from build123d import *

# Parameters (mm, degrees)
F0_W      = 160.02
F0_H      = 160.02
F1_DEPTH  = 61.214
F3_DEPTH  = 58.42
F4_R      = 3.937
F5_DEPTH  = 6.35
F7_DEPTH  = 6.35
F8_R      = 1.7018
F9_DEPTH  = 6.35
F11_R     = 6.35
F12_DEPTH = 6.35
F13_R     = 3.175
F14_DEPTH = 6.35
F15_R     = 6.35
F16_DEPTH = 6.35
F17_R     = 6.35
F18_DEPTH = 6.35
F19_R     = 3.81
F20_DEPTH = 6.35
F23_DEPTH = 6.35
F24_W     = 12.7
F24_H     = 12.7
F24_R     = 1.8288
F25_DEPTH = 6.35


with BuildPart() as f1:
    # F0 (on Top) → F1 (new body)
    with BuildSketch(Plane.XY):
        with Locations((80.01, 80.01)):
            Rectangle(F0_W, F0_H)
    extrude(amount=-F1_DEPTH)

    # F2 (on face) → F3 (cut)
    with BuildSketch(Plane.XY):
        Polygon((142.24, 154.305), (17.78, 154.305), (17.78, 135.89), (5.08, 135.89), (5.08, 24.13), (17.78, 24.13), (17.78, 5.715), (142.24, 5.715), (142.24, 24.13), (154.94, 24.13), (154.94, 135.89), (142.24, 135.89), align=None)
    extrude(amount=-F3_DEPTH, mode=Mode.SUBTRACT)

    # F4 (on face) → F5 (cut)
    with BuildSketch(Plane.XZ):
        with Locations((32.7025, -45.974)):
            Circle(F4_R)
        with Locations((127.3429, -45.974)):
            Circle(F4_R)
    extrude(amount=-F5_DEPTH, mode=Mode.SUBTRACT)

    # F6 (on face) → F7 (cut)
    with BuildSketch(Plane.XZ):
        with BuildLine():
            Line((81.1022, -35.9791), (61.1378, -35.9791))
            ThreePointArc((61.1378, -35.9791), (58.318, -37.1471), (57.15, -39.9669))
            Line((57.15, -39.9669), (57.15, -51.9811))
            ThreePointArc((57.15, -51.9811), (58.318, -54.8009), (61.1378, -55.9689))
            Line((61.1378, -55.9689), (81.1022, -55.9689))
            ThreePointArc((81.1022, -55.9689), (83.922, -54.8009), (85.09, -51.9811))
            Line((85.09, -51.9811), (85.09, -39.9669))
            ThreePointArc((85.09, -39.9669), (83.922, -37.1471), (81.1022, -35.9791))
        make_face()
    extrude(amount=-F7_DEPTH, mode=Mode.SUBTRACT)

    # F8 (on face) → F9 (cut)
    with BuildSketch(Plane.XZ):
        with Locations((51.1302, -45.974)):
            Circle(F8_R)
        with Locations((91.0082, -45.974)):
            Circle(F8_R)
    extrude(amount=-F9_DEPTH, mode=Mode.SUBTRACT)

    # F11 (on face) → F12 (cut)
    with BuildSketch(Plane.XZ):
        with Locations((32.6898, -26.924)):
            Circle(F11_R)
        with Locations((127.3302, -26.924)):
            Circle(F11_R)
    extrude(amount=-F12_DEPTH, mode=Mode.SUBTRACT)

    # F13 (on face) → F14 (cut)
    with BuildSketch(Plane.XZ):
        with Locations((32.6898, -10.414)):
            Circle(F13_R)
        with Locations((127.3302, -10.414)):
            Circle(F13_R)
    extrude(amount=-F14_DEPTH, mode=Mode.SUBTRACT)

    # F15 (on face) → F16 (cut)
    with BuildSketch(Plane.XZ):
        with Locations((71.12, -16.764)):
            Circle(F15_R)
    extrude(amount=-F16_DEPTH, mode=Mode.SUBTRACT)

    # F17 (on face) → F18 (cut)
    with BuildSketch(Plane.XZ):
        with Locations((106.68, -26.924)):
            Circle(F17_R)
    extrude(amount=-F18_DEPTH, mode=Mode.SUBTRACT)

    # F19 (on face) → F20 (cut)
    with BuildSketch(Plane.XZ):
        with Locations((106.68, -10.414)):
            Circle(F19_R)
    extrude(amount=-F20_DEPTH, mode=Mode.SUBTRACT)

    # F22 (on face) → F23 (cut)
    with BuildSketch(Plane(origin=(0, 160.02, 0), x_dir=(-1, 0, 0), z_dir=(0, 1, 0))):
        with BuildLine():
            ThreePointArc((-139.419261, -17.800688), (-140.943261, -19.324688), (-139.419261, -20.848688))
            Line((-139.419261, -20.848688), (-137.312171, -20.848688))
            ThreePointArc((-137.312171, -20.848688), (-136.789713, -21.038847), (-136.511719, -21.520347))
            Line((-136.511719, -21.520347), (-136.061514, -24.07359))
            ThreePointArc((-136.061514, -24.07359), (-135.345498, -25.318244), (-133.998495, -25.815663))
            Line((-133.998495, -25.815663), (-97.890658, -26.040951))
            ThreePointArc((-97.890658, -26.040951), (-96.527424, -25.551986), (-95.801333, -24.298877))
            Line((-95.801333, -24.298877), (-95.311403, -21.520347))
            ThreePointArc((-95.311403, -21.520347), (-95.033409, -21.038847), (-94.510951, -20.848688))
            Line((-94.510951, -20.848688), (-92.378461, -20.848688))
            ThreePointArc((-92.378461, -20.848688), (-90.854461, -19.324688), (-92.378461, -17.800688))
            Line((-92.378461, -17.800688), (-93.686869, -17.800688))
            ThreePointArc((-93.686869, -17.800688), (-94.30951, -17.510346), (-94.487321, -16.846747))
            Line((-94.487321, -16.846747), (-94.211744, -15.283873))
            ThreePointArc((-94.211744, -15.283873), (-94.672941, -13.562664), (-96.287916, -12.809588))
            Line((-96.287916, -12.809588), (-135.535206, -12.809588))
            ThreePointArc((-135.535206, -12.809588), (-137.150181, -13.562664), (-137.611378, -15.283873))
            Line((-137.611378, -15.283873), (-137.335801, -16.846747))
            ThreePointArc((-137.335801, -16.846747), (-137.513612, -17.510346), (-138.136253, -17.800688))
            Line((-138.136253, -17.800688), (-139.419261, -17.800688))
        make_face()
        with BuildLine():
            ThreePointArc((-139.446, -43.6499), (-140.97, -45.1739), (-139.446, -46.6979))
            Line((-139.446, -46.6979), (-137.33891, -46.6979))
            ThreePointArc((-137.33891, -46.6979), (-136.816452, -46.888059), (-136.538458, -47.369559))
            Line((-136.538458, -47.369559), (-136.088253, -49.922801))
            ThreePointArc((-136.088253, -49.922801), (-135.372237, -51.167456), (-134.025234, -51.664875))
            Line((-134.025234, -51.664875), (-97.917397, -51.890162))
            ThreePointArc((-97.917397, -51.890162), (-96.554163, -51.401198), (-95.828072, -50.148088))
            Line((-95.828072, -50.148088), (-95.338142, -47.369559))
            ThreePointArc((-95.338142, -47.369559), (-95.060148, -46.888059), (-94.53769, -46.6979))
            Line((-94.53769, -46.6979), (-92.4052, -46.6979))
            ThreePointArc((-92.4052, -46.6979), (-90.8812, -45.1739), (-92.4052, -43.6499))
            Line((-92.4052, -43.6499), (-93.713608, -43.6499))
            ThreePointArc((-93.713608, -43.6499), (-94.336249, -43.359558), (-94.51406, -42.695959))
            Line((-94.51406, -42.695959), (-94.238483, -41.133085))
            ThreePointArc((-94.238483, -41.133085), (-94.69968, -39.411875), (-96.314655, -38.6588))
            Line((-96.314655, -38.6588), (-135.561945, -38.6588))
            ThreePointArc((-135.561945, -38.6588), (-137.17692, -39.411875), (-137.638117, -41.133085))
            Line((-137.638117, -41.133085), (-137.36254, -42.695959))
            ThreePointArc((-137.36254, -42.695959), (-137.540351, -43.359558), (-138.162992, -43.6499))
            Line((-138.162992, -43.6499), (-139.446, -43.6499))
        make_face()
    extrude(amount=-F23_DEPTH, mode=Mode.SUBTRACT)

    # F24 (on face) → F25 (cut)
    with BuildSketch(Plane(origin=(0, 160.02, 0), x_dir=(-1, 0, 0), z_dir=(0, 1, 0))):
        with Locations((-45.72, -45.339)):
            Rectangle(F24_W, F24_H)
        with Locations((-60.706, -45.339)):
            Circle(F24_R)
        with Locations((-30.7086, -45.339)):
            Circle(F24_R)
    extrude(amount=-F25_DEPTH, mode=Mode.SUBTRACT)


solid = f1.part
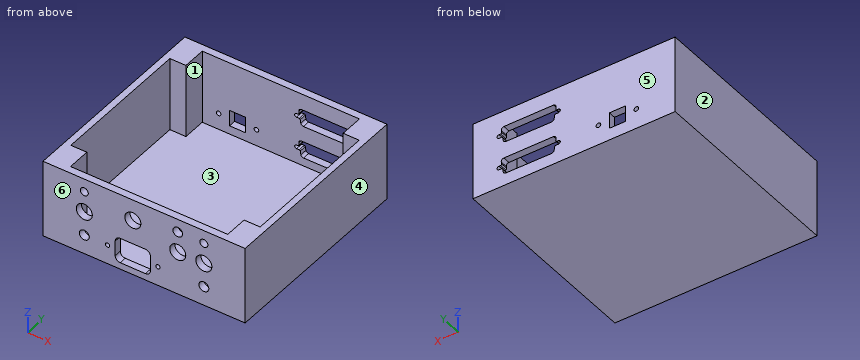
Work out the finished part from the listing and answer in its coordinate system (mm). Face numbers are marked on the shaded views. A direction names the side the tool comes from. Round coordinates to 2 decimals unless told otherwise and drop trailing zeros. Write each loop counter-clockwise with the first axis right and the second up, starting at its lowest first coordinate (ties: lowest second). Pieces come first, ordered by that corner, then holes.
1) A tool of negligible diameter and unlimited length cuts with its end or side. For the marked faces 1 and 2, from which of +Z, -Z, +X, -X, +Y, -Y can it reach the whole face along a straight path? Write none if from no direction.
2) Straight lines are drawn through the part: line 1 (X direction, y = 87, z = -51); line 2 (Y direction, x = 78.5, z = -22.5) (3 decimals); line 3 (X direction, y = 152, z = -50.5). For each, find the intervals that lie inside material, in ascending order.
3) A cutting plane is placed at B-B (x = 71.12). Give the vertices of the cut face in (y, z) (3 decimals).
4) Given pin 1 Ø8 at (x, y) = (92.5, 53) entering from +Z, flat-ended and moving along its own axis, determine where the tip first touches the part or whether it passes through.
5) A cutting plane is placed at C-C (y = 32.5). Give the vertices of the cut face in (x, z).
6) A cutting plane is placed at D-D (x = 148). Give the vertices of the cut face in (y, z).
7) The mould has two halves that part along Y. Classify the marked faces 3, 4, 5 and 6: pulls with the +Y half, pulls with the -Y half, needs draft (parallel to the pull), parting line crosses it, or undercut.
8) A cutting plane is placed at A-A (x = 45). Give the vertices of the cut face in (y, z) (3 decimals).
Completed:
1. face 1: +Z
1. face 2: +Z, -Z, -X, +Y, -Y
2. line 1: x = 0 to 5.08, 154.94 to 160.02
2. line 2: y = 0 to 5.715, 154.305 to 160.02
2. line 3: x = 0 to 17.78, 142.24 to 160.02
3. outline: (0, -61.214) - (160.02, -61.214) - (160.02, 0) - (154.305, 0) - (154.305, -58.42) - (5.715, -58.42) - (5.715, -55.969) - (0, -55.969) - close; (0, -35.979) - (5.715, -35.979) - (5.715, -23.114) - (0, -23.114) - close; (0, -10.414) - (5.715, -10.414) - (5.715, 0) - (0, 0) - close
4. pin 1: stops at z = -58.42
5. outline: (0, -61.21) - (160.02, -61.21) - (160.02, 0) - (154.94, 0) - (154.94, -58.42) - (5.08, -58.42) - (5.08, 0) - (0, 0) - close
6. outline: (0, -61.21) - (160.02, -61.21) - (160.02, 0) - (135.89, 0) - (135.89, -58.42) - (24.13, -58.42) - (24.13, 0) - (0, 0) - close
7. face 3: undercut
7. face 4: needs draft
7. face 5: pulls with the +Y half
7. face 6: pulls with the -Y half
8. outline: (0, -61.214) - (160.02, -61.214) - (160.02, -51.689) - (154.305, -51.689) - (154.305, -58.42) - (5.715, -58.42) - (5.715, 0) - (0, 0) - close; (154.305, -38.989) - (160.02, -38.989) - (160.02, 0) - (154.305, 0) - close
